Here's how the part is built. I have some questions about the finished solid (model axes, mm). A direction names the side the tool comes from. Coordinates: 2 decimals unless noted, no trailing zeros. Write each loop counter-clockwise with the first axis right and the second up, starting at its lowest first coordinate (ties: lowest second). Pieces come first, ordered by that corner, then holes. Notation, with made-up numbers: (11.25, -17.5) -> (38.25, -17.5) arc R27 ccw to (38.25, 8.5) -> close; hole circle Ø10 at (64, -35.75). An arc over 180 degrees is marked (long way). Put each result on its own line as item: value. Start each with the question number.
Item 1: On a 3-axis mill with a long thin cutter (end or side, diameter ignored), from which of +Z, -Z, +X, -X, +Y, -Y can I reach the whole of each face in a straight line? I mean faces 5 (the face through (23, 6, 12)), 6 (the face through (-32, -14, 4)), 7 (the face through (-32, -14, 21)), 8 (the face through (-6.9, -16.69, 12.68)), 9 (the face through (3.5, -12, 22)). Say none if no direction works.
Item 2: For pin 1 (1.5 mm diameter, centred on y = -4.5, z = 19, fed in from -X); pin 2 (1.5 mm diameter, centred on x = 10.5, z = 5.5, fed in from +Y); pin 3 (2 mm diameter, centred on y = -12.5, z = 1.5, fed in from -X), each with a flat end and sliding along its axis, tell me the tip position at first contact or that it passes through.
Item 3: If we mould it in two halves opening along X, with no side actions, what happens to faces 1 (the face through (0, -11, 18)), 2 (the face through (-29, -14, 23)), 3 (the face through (-16, -14, 25)), 4 (the face through (7.098, -16.782, 12.675))? For each: released by +X, released by -X, zero draft, split by the parting line, or undercut.
Item 4: I want a section at A-A, the plane y = 17. List the corners of the cut face in (x, z) for me, then the cut area to 4 significant figures.
Item 5: I need wall thicknesses on line 1 (X direction, y = -1, z = 19.5); line 2 (Y direction, x = -26, z = 11.5); line 3 (X direction, y = -14.5, z = 15). Which ranges of each line are inside material? Lowest first, please. Write a range as [from, to].
Item 6: I want a section at B-B, the plane z = 8.25. List the corners of the cut face in (x, y) for me.
Item 7: I want a section at C-C, the plane x = -19. List the corners of the cut face in (y, z) for me.
Item 8: I want a section at D-D, the plane z = 2. List the corners of the cut face in (x, y) for me, then the cut area to 3 significant figures.
from build123d import *

# Parameters (mm, degrees)
EXTRUDE_1_DEPTH     = 25
CUT_EXTRUDE_1_DEPTH = 48.434164903
SKETCH_3_W          = 6
SKETCH_3_H          = 4
SKETCH_3_W_2        = 7
SKETCH_3_H_2        = 7
CUT_EXTRUDE_2_DEPTH = 52.322509681


with BuildPart() as part:
    # Эскиз1 → Бобышка-Вытянуть1 (new body)
    with BuildSketch(Plane.XY):
        Polygon((23, -8), (-35, -8), (-35, -20), (35, -20), (35, 20), (23, 20), align=None)
    extrude(amount=EXTRUDE_1_DEPTH)

    # Эскиз2 → Вырез-Вытянуть1 (cut, through all)
    with BuildSketch(Plane.XY.offset(25)):
        Polygon((35, -20), (35, -11), (26, -20), align=None)
        Polygon((-14, -20), (14, -20), (0, -13.471692786), align=None)
        Polygon((23, 20), (29, 12), (35, 20), align=None)
    extrude(amount=-CUT_EXTRUDE_1_DEPTH, mode=Mode.SUBTRACT)

    # Эскиз3 → Вырез-Вытянуть2 (cut, through all)
    with BuildSketch(Plane(origin=(0, -8, 0), x_dir=(1, 0, 0), z_dir=(0, 1, 0))):
        with Locations((-32, -23)):
            Rectangle(SKETCH_3_W, SKETCH_3_H)
        with Locations((-32, -2)):
            Rectangle(SKETCH_3_W, SKETCH_3_H)
        with Locations((0, -21.5)):
            Rectangle(SKETCH_3_W_2, SKETCH_3_H_2)
    extrude(amount=-CUT_EXTRUDE_2_DEPTH, mode=Mode.SUBTRACT)


solid = part.part
Calculated:
1. face 5: +Z, -Z, -X, +Y
1. face 6: -Z, -X, +Y, -Y
1. face 7: +Z, -X, +Y, -Y
1. face 8: +Z, -Z, -Y
1. face 9: +Z, +Y, -Y
2. pin 1: stops at x = 23
2. pin 2: stops at y = -8
2. pin 3: stops at x = -29
3. face 1: undercut
3. face 2: released by -X
3. face 3: zero draft
3. face 4: undercut
4. outline: (23, 0) -> (25.25, 0) -> (25.25, 25) -> (23, 25) -> close; (32.75, 0) -> (35, 0) -> (35, 25) -> (32.75, 25) -> close
4. area: 112.5 mm2
5. line 1: x = [23, 35]
5. line 2: y = [-20, -8]
5. line 3: x = [-35, -2.21], [2.21, 31.5]
6. outline: (-35, -20) -> (-14, -20) -> (0, -13.47) -> (14, -20) -> (26, -20) -> (35, -11) -> (35, 20) -> (29, 12) -> (23, 20) -> (23, -8) -> (-35, -8) -> close
7. outline: (-20, 0) -> (-8, 0) -> (-8, 25) -> (-20, 25) -> close
8. outline: (-29, -20) -> (-14, -20) -> (0, -13.47) -> (14, -20) -> (26, -20) -> (35, -11) -> (35, 20) -> (29, 12) -> (23, 20) -> (23, -8) -> (-29, -8) -> close
8. area: 924 mm2
